For this review, use the dimensioned drawing (mm, ordinates from the lowest corner) and the shaded views. A direction names the side the tool comes from. Coordinates: 2 decimals unless noted, no trailing zeros. Loops run counter-clockwise (first coordinate to the right, second up) from the corner with the lowest first, then second, coordinate; pieces in that order, holes last. Notation, with made-up numbers: M 67,-34 L 109,-34 A22 ccw 109,-11 Z; hole C 81,-18.75 d2. An arc over 180 degrees is marked long. Write item = value, one per line.
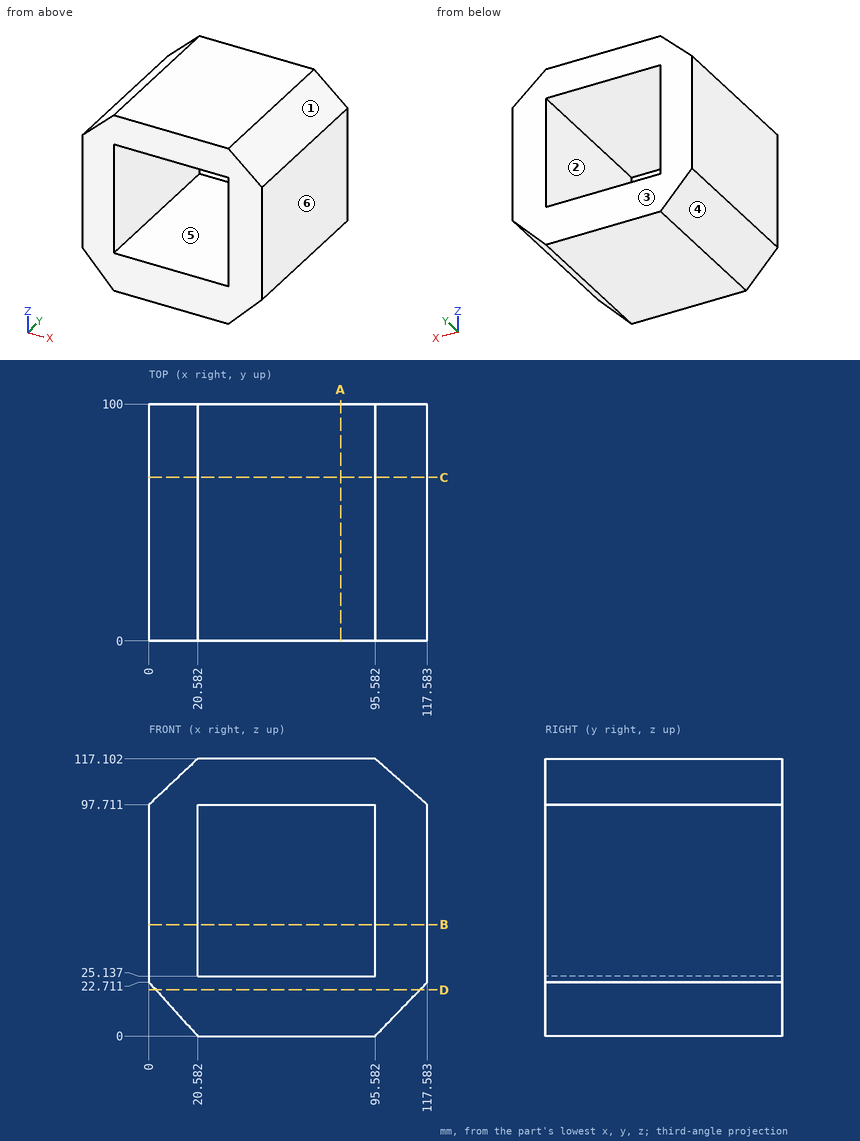
Q1. Add section A-A (x = 81). Write out the cut boundary in (y, z).
Solved:
outline = M 0,0 L 100,0 L 100,25.14 L 0,25.14 Z; M 0,97.71 L 100,97.71 L 100,117.1 L 0,117.1 Z
Q2. Machinability: for the marked faces 1 and 2, which of the approach directions +Z, -Z, +X, -X, +Y, -Y give a long, thin tool a straight path to every point of the face, cutting with its end or side? Answer none if there is none.
Solved:
face_1 = +Z, +X, +Y, -Y
face_2 = +Y, -Y
Q3. Add section C-C (y = 69). Write out the cut boundary in (x, z), and give its area (3 significant figures).
Solved:
outline = M 0,22.71 L 20.58,0 L 95.58,0 L 117.58,22.71 L 117.58,97.71 L 95.58,117.1 L 20.58,117.1 L 0,97.71 Z; hole M 20.58,25.14 L 95.58,25.14 L 95.58,97.71 L 20.58,97.71 Z
area = 7,430 mm²
Q4. Add section B-B (z = 47). Write out the cut boundary in (x, y).
Solved:
outline = M 0,0 L 20.58,0 L 20.58,100 L 0,100 Z; M 95.58,0 L 117.58,0 L 117.58,100 L 95.58,100 Z
Q5. Add section D-D (z = 19.5). Write out the cut boundary in (x, y), and give its area (3 significant figures).
Solved:
outline = M 2.91,0 L 114.47,0 L 114.47,100 L 2.91,100 Z
area = 11,200 mm²
Q6. For line 1 along Z through (x, y) = (39, 72); line 2 along X through (y, z) = (5, 47); line 3 along Z through (x, y) = (105, 33), list the stretches that pass through material, from the lowest coordinate up.
Solved:
line_1 = 0 to 25.14, 97.71 to 117.1
line_2 = 0 to 20.58, 95.58 to 117.58
line_3 = 9.72 to 108.8
Q7. Draft analysis for pull direction X (two halves, no side actions). For the marked faces 3, 4, 5 and 6, state which applies: +X half, -X half, draft (parallel to the pull), parting line (faces both ways), or undercut.
Solved:
face_3 = draft
face_4 = -X half
face_5 = undercut
face_6 = +X half
